Could you check a few things on this drawing? It's one solid part, dimensions in mm from its lowest x, y, z. Give positions to 0.01 mm unless a question says otherwise; leave off trailing zeros. Order: outer loops, then holes, each group sorted by start corner. A loop starts at its lowest first (then second) coordinate and runs counter-clockwise, first axis right, second up. Notation, with made-up numbers: (-21.5, -25) -> (-1.5, -25) arc R19 ccw to (-1.5, 12) -> close; hole circle Ø7 at (-3.5, 54.25). An arc over 180 degrees is marked (long way). Answer as CSV lines item,"result".
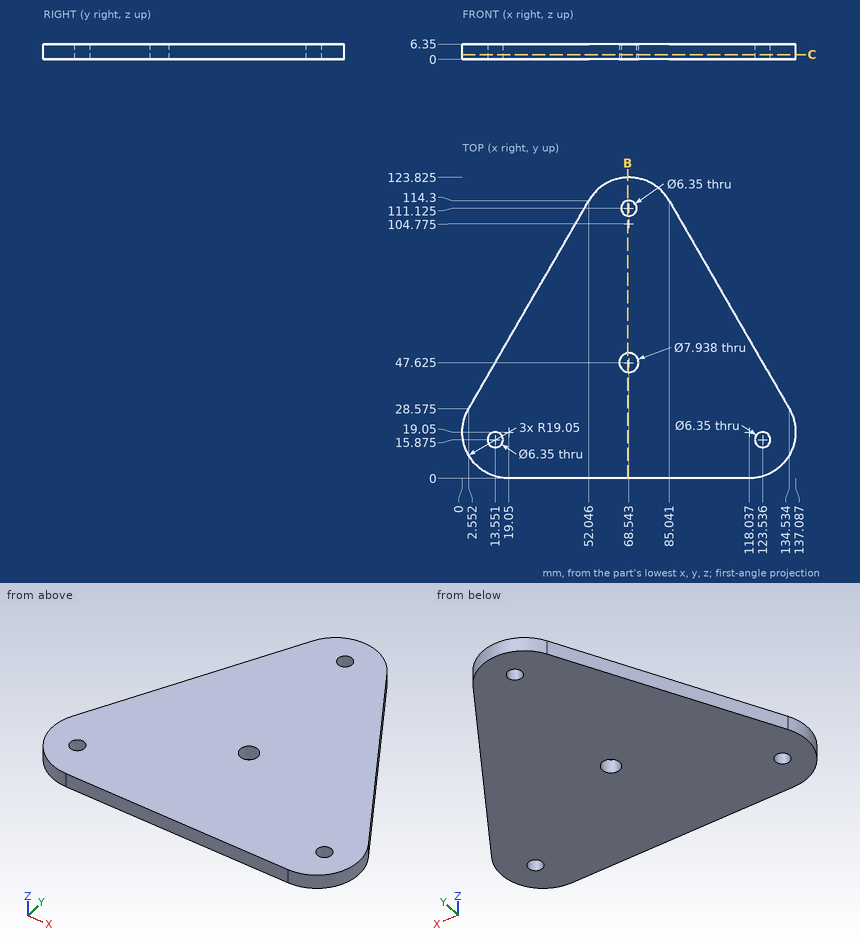
Item 1: For pin 1 (10 mm diameter, centred on x = 123.54, y = 15.88, fed in from +Z); pin 2 (5 mm diameter, centred on x = 68.54, y = 47.62, fed in from -Z); pin 3 (1 mm diameter, centred on y = 28, z = 4, fed in from -X); pin 4 (1.5 mm diameter, centred on y = 47, z = 0.5, fed in from -X), each with a flat end and sliding along its axis, tell me the tip position at first contact or that it passes through.
Numbers:
pin 1,"stops at z = 6.35"
pin 2,"passes through"
pin 3,"stops at x = 1.98"
pin 4,"stops at x = 12.76"
Item 2: Please list where these lines run through material, in increasing order: line 1 along Y through (x, z) = (66.5, 4.25) (1 decimal); line 2 along X through (y, z) = (50, 5.75) (1 decimal); line 3 along Y through (x, z) = (101, 2) (1 decimal).
Numbers:
line 1,"y = 0 to 44.2, 51 to 108.7, 113.6 to 123.7"
line 2,"x = 14.9 to 65.4, 71.7 to 122.2"
line 3,"y = 0 to 86.7"
Item 3: Imagine slicing it at B-B, the plane x = 68. Please give me the cut outline in (y, z).
Numbers:
outline,"(0, 0) -> (43.69, 0) -> (43.69, 6.35) -> (0, 6.35) -> close; (51.56, 0) -> (108, 0) -> (108, 6.35) -> (51.56, 6.35) -> close; (114.25, 0) -> (123.82, 0) -> (123.82, 6.35) -> (114.25, 6.35) -> close"
Item 4: Imagine slicing it at C-C, the plane z = 2. Give the number of separate pieces and of enclosed holes in the cut face, then the cut area to 3 significant figures.
Numbers:
separate pieces,"1"
enclosed holes,"4"
area,"10,900 mm²"
